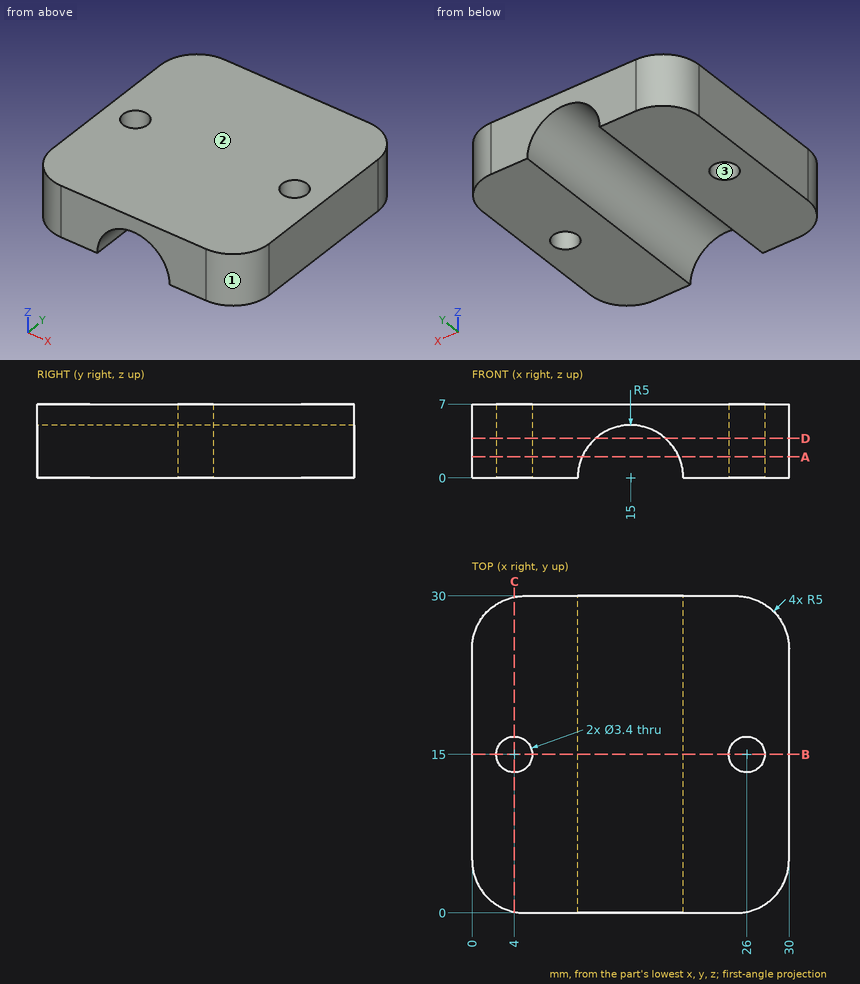
Job drawing, mm, ordinate dimensions from the low corner. One solid piece. Round coordinates to 2 decimals unless told otherwise and drop trailing zeros. Order: outer loops, then holes, each group sorted by start corner. A loop starts at its lowest first (then second) coordinate and runs counter-clockwise, first axis right, second up. Notation, with made-up numbers: (35, -20) - (79, -20) arc R31 cw to (79, 10) - close; hole circle Ø1 at (53.5, 73). An arc over 180 degrees is marked (long way). Use CSV: the item, a comma, the result in double quotes. Start each with the question number.
1) Saw through at B-B (y = 15). List the corners of the cut face in (x, z).
2) Pin check, flat tip, straight feed: pin 1 Ø4 at (x, y) = (15.5, 26.5) entering from -Z. Stop position of the tip, or through.
3) Wall check: L1, parallel to X at y = 14, z = 2; L2, parallel to Y at x = 3, z = 1.5; L3, parallel to Y at x = 4, z = 2.5. Give the ranges that are in metal, low to high. Write a range as [from, to].
4) Saw through at D-D (z = 3.75). List the corners of the cut face in (x, y), and give its area (3 significant figures).
5) Saw through at A-A (z = 2). List the corners of the cut face in (x, y), and give its area (3 significant figures).
6) Two-plate mould, pull along X, no slides. Class the marked faces 1, 2 and 3: pulls with the +X half, pulls with the -X half, needs draft (parallel to the pull), parting line crosses it, or undercut.
7) Saw through at C-C (x = 4). List the corners of the cut face in (y, z).
Values follow:
1,outline,"(0, 0) - (2.3, 0) - (2.3, 7) - (0, 7) - close; (5.7, 0) - (10, 0) arc R5 cw to (20, 0) - (24.3, 0) - (24.3, 7) - (5.7, 7) - close; (27.7, 0) - (30, 0) - (30, 7) - (27.7, 7) - close"
2,pin 1,"stops at z = 4.33"
3,L1,"x = [0, 2.63], [5.37, 10.42], [19.58, 24.63], [27.37, 30]"
3,L2,"y = [0.42, 13.63], [16.37, 29.58]"
3,L3,"y = [0.1, 13.3], [16.7, 29.9]"
4,outline,"(0, 5) arc R5 ccw to (5, 0) - (11.69, 0) - (11.69, 30) - (5, 30) arc R5 ccw to (0, 25) - close; (18.31, 0) - (25, 0) arc R5 ccw to (30, 5) - (30, 25) arc R5 ccw to (25, 30) - (18.31, 30) - close; hole circle Ø3.4 at (4, 15); hole circle Ø3.4 at (26, 15)"
4,area,"662 mm2"
5,outline,"(0, 5) arc R5 ccw to (5, 0) - (10.42, 0) - (10.42, 30) - (5, 30) arc R5 ccw to (0, 25) - close; (19.58, 0) - (25, 0) arc R5 ccw to (30, 5) - (30, 25) arc R5 ccw to (25, 30) - (19.58, 30) - close; hole circle Ø3.4 at (4, 15); hole circle Ø3.4 at (26, 15)"
5,area,"585 mm2"
6,face 1,"pulls with the +X half"
6,face 2,"needs draft"
6,face 3,"undercut"
7,outline,"(0.1, 0) - (13.3, 0) - (13.3, 7) - (0.1, 7) - close; (16.7, 0) - (29.9, 0) - (29.9, 7) - (16.7, 7) - close"
